Input: part model. Units: mm. Frame: model coordinates. Round coordinates to 2 decimals unless told otherwise and drop trailing zeros. Loops run counter-clockwise (first coordinate to the right, second up) from the corner with the lowest first, then second, coordinate; pieces in that order, holes last.
(1) Cut plane A-A, the plane z = 58.5. Output: boundary loops of the cut face in (x, y) (1 decimal).
(2) Cut plane B-B, the plane y = 27. Output: boundary loops of the cut face in (x, z).
(3) First-contact query: pin 1 Ø4 at (x, z) = (50, 43) entering from +Y; pin 2 Ø2 at (x, z) = (56, 34) entering from -Y; pin 3 Ø12 at (y, z) = (-41, 38) entering from +X. Flat tips, straight axial feed; report the tip coordinate or a pass-through.
(4) Cut plane C-C, the plane x = 2.5. Output: boundary loops of the cut face in (y, z).
(5) Cut plane D-D, the plane z = 18.5. Output: boundary loops of the cut face in (x, y), and give its area (3 significant figures).
(6) Line query: line 1 (Z direction, x = 20.5, y = 13); line 2 (X direction, y = -1, z = 30.5); line 3 (X direction, y = -11.5, z = 38.5). Output: solid intervals per line, ascending.
from build123d import *

# Parameters (mm, degrees)
F1_DEPTH = 50
F2_DEPTH = 65
F3_R     = 10


with BuildPart() as f1:
    # F0 (on Top) → F1 (new body)
    with BuildSketch(Plane.XY):
        with BuildLine():
            Line((18.428938438, -31.0235001472), (72.1632169215, 0.8963575571))
            Line((72.1632169215, 0.8963575571), (-36.8578768761, 62.0470002943))
            Line((-36.8578768761, 62.0470002943), (-22.982297547, 38.6886805081))
            ThreePointArc((-22.982297547, 38.6886805081), (-12.9289992244, 38.7823343206), (-7.8751203144, 30.0911959508))
            ThreePointArc((-7.8751203144, 30.0911959508), (-9.1839819445, 25.1450748608), (-12.7679430817, 21.4937113934))
            Line((-12.7679430817, 21.4937113934), (0, 0))
            Line((0, 0), (4.1072919863, -6.9142655162))
            ThreePointArc((4.1072919863, -6.9142655162), (14.160590309, -6.8206117038), (19.214469219, -15.5117500736))
            ThreePointArc((19.214469219, -15.5117500736), (17.9056075888, -20.4578711635), (14.3216464517, -24.1092346309))
            Line((14.3216464517, -24.1092346309), (18.428938438, -31.0235001472))
        make_face()
        with BuildLine():
            Line((-35.3053400455, -62.9433578514), (18.428938438, -31.0235001472))
            Line((18.428938438, -31.0235001472), (14.3216464517, -24.1092346309))
            ThreePointArc((14.3216464517, -24.1092346309), (0.6169846617, -20.6189273063), (4.1072919863, -6.9142655162))
            Line((4.1072919863, -6.9142655162), (0, 0))
            Line((0, 0), (-12.7679430817, 21.4937113934))
            ThreePointArc((-12.7679430817, 21.4937113934), (-26.4726048717, 24.9840187181), (-22.982297547, 38.6886805081))
            Line((-22.982297547, 38.6886805081), (-36.8578768761, 62.0470002943))
            Line((-36.8578768761, 62.0470002943), (-35.3053400455, -62.9433578514))
        make_face()
    extrude(amount=F1_DEPTH)

    # F0 (on Top) → F2 (join)
    with BuildSketch(Plane.XY):
        with BuildLine():
            ThreePointArc((-7.8751203144, 30.0911959508), (-12.9289992244, 38.7823343206), (-22.982297547, 38.6886805081))
            Line((-22.982297547, 38.6886805081), (-12.7679430817, 21.4937113934))
            ThreePointArc((-12.7679430817, 21.4937113934), (-9.1839819445, 25.1450748608), (-7.8751203144, 30.0911959508))
        make_face()
        with BuildLine():
            Line((-12.7679430817, 21.4937113934), (-22.982297547, 38.6886805081))
            ThreePointArc((-22.982297547, 38.6886805081), (-26.4726048717, 24.9840187181), (-12.7679430817, 21.4937113934))
        make_face()
        with BuildLine():
            ThreePointArc((4.1072919863, -6.9142655162), (0.6169846617, -20.6189273063), (14.3216464517, -24.1092346309))
            Line((14.3216464517, -24.1092346309), (4.1072919863, -6.9142655162))
        make_face()
        with BuildLine():
            Line((4.1072919863, -6.9142655162), (14.3216464517, -24.1092346309))
            ThreePointArc((14.3216464517, -24.1092346309), (17.9056075888, -20.4578711635), (19.214469219, -15.5117500736))
            ThreePointArc((19.214469219, -15.5117500736), (14.160590309, -6.8206117038), (4.1072919863, -6.9142655162))
        make_face()
    extrude(amount=F2_DEPTH)

    # F3
    f3_edges = [f1.edges().sort_by_distance(p)[0] for p in [
        (-27.87512, 30.091196, 65),
        (4.107292, -6.914266, 65),
    ]]
    fillet(f3_edges, radius=F3_R)


solid = f1.part
Reported:
1. outline: circle Ø18.7 at (-17.9, 30.1); circle Ø18.7 at (9.2, -15.5)
2. outline: (-36.42, 0) - (25.62, 0) - (25.62, 50) - (-8.36, 50) - (-8.36, 55) arc R9.51 ccw to (-27.39, 55) - (-27.39, 50) - (-36.42, 50) - close
3. pin 1: stops at y = 14.45
3. pin 2: stops at y = -9.3
3. pin 3: stops at x = 11.73
4. outline: (-40.49, 0) - (39.97, 0) - (39.97, 50) - (-8.1, 50) - (-8.1, 55) arc R7.41 ccw to (-22.92, 55) - (-22.92, 50) - (-40.49, 50) - close
5. outline: (-36.86, 62.05) - (-35.31, -62.94) - (72.16, 0.9) - close
5. area: 6,770 mm2
6. line 1: z = 0 to 50
6. line 2: x = -36.07 to 68.97
6. line 3: x = -35.94 to 51.3
